Geometry: final body of the model. Coordinates: model frame, mm. Face numbers are marked on the shaded views. A direction names the side the tool comes from. Round coordinates to 2 decimals unless told otherwise and drop trailing zeros. Order: outer loops, then holes, each group sorted by start corner. A loop starts at its lowest first (then second) coordinate and runs counter-clockwise, first axis right, second up. Notation, with made-up numbers: (4, 68) -> (38, 68) arc R18 ccw to (38, 72) -> close; hole circle Ø3 at (73, 59). An arc over 180 degrees is marked (long way). Put each result on its own line as item: value.
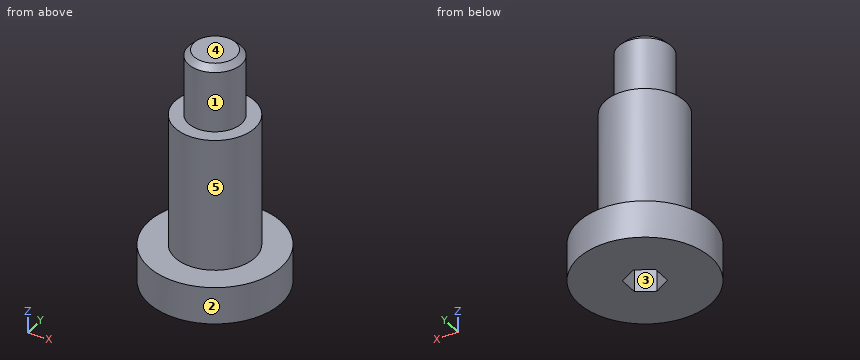
Autodesk Inventor part; units mm, degrees
ref_plane "YZ Plane" through (0, 0, 0) normal (1, 0, 0) x (0, 1, 0)
ref_plane "XZ Plane" through (0, 0, 0) normal (0, 1, 0) x (-1, 0, 0)
ref_plane "XY Plane" through (0, 0, 0) normal (0, 0, 1) x (1, 0, 0)
sketch "Sketch1" plane through (0, 0, 0) normal (0, 1, 0) x (-1, 0, 0)
  line L0 (0, 0) -> (0, 17.8)
  line L1 (0, 17.8) -> (-2, 17.8)
  line L2 (-2, 17.8) -> (-2, 12.8)
  line L3 (-2, 12.8) -> (-3, 12.8)
  line L4 (-3, 12.8) -> (-3, 2.8)
  line L5 (-3, 2.8) -> (-5, 2.8)
  line L6 (-5, 2.8) -> (-5, 0)
  line L7 (-5, 0) -> (0, 0)
  dimension "d0" = 10
  dimension "d1" = 6
  dimension "d2" = 4
  dimension "d3" = 5
  dimension "d4" = 10
  dimension "d5" = 2.8
revolve "Revolution1" add sketch "Sketch1" angle 360 about axis through (0, 0, 0) along (0, 0, 1)
thread "Thread1"
sketch "Sketch2" plane through (0, 0, 0) normal (0, 0, -1) x (-1, 0, 0)
  line L0 (0, 1.4434) -> (1.25, 0.7217)
  line L1 (1.25, 0.7217) -> (1.25, -0.7217)
  line L2 (1.25, -0.7217) -> (0, -1.4434)
  line L3 (0, -1.4434) -> (-1.25, -0.7217)
  line L4 (-1.25, -0.7217) -> (-1.25, 0.7217)
  line L5 (-1.25, 0.7217) -> (0, 1.4434)
  point P0 (0, 0)
  point P1 (0, 0)
  dimension "d9" = 2.5
extrude "Extrusion1" cut sketch "Sketch2" against normal blind 2
chamfer "Chamfer1" distance 0.43 angle 45 1 edges at (-2, 0, 17.8)
properties part number "DBTSY4-10-5-DHC" material "Stainless Steel AISI 304"
1. Cut plane B-B on z = 16.5. Return loops of the section in (x, y).
Ans:
outline: circle Ø4 at (0, 0)
2. Material intervals for probe 1 along Z at (x, y) = (-2.25, -4); probe 2 along Z at (x, y) = (1.5, -1.5); probe 3 along X at (y, z) = (-2, 11), sorted ascending.
Ans:
probe 1: 0 to 2.8
probe 2: 0 to 12.8
probe 3: -2.24 to 2.24
3. Set-up query: the marked faces 1 and 2. Return all of +Z, -Z, +X, -X, +Y, -Y with unobstructed straight access to the full face (end or side cutting, diameter ignored); none if empty.
Ans:
face 1: +Z
face 2: +Z, -Z
4. Cut plane C-C on x = 2.5. Return loops of the section in (y, z), and give its area (3 significant figures).
Ans:
outline: (-4.33, 0) -> (4.33, 0) -> (4.33, 2.8) -> (1.66, 2.8) -> (1.66, 12.8) -> (-1.66, 12.8) -> (-1.66, 2.8) -> (-4.33, 2.8) -> close
area: 57.4 mm²
5. Contact query for flat-ended pins moving along their axis: P1, Ø2, axis at y = 2, z = 9.5, coming from the +X side; P2, Ø4, axis at x = -2, y = -3, coming from the +Z side; P3, Ø3, axis at x = 1.5, z = 13.5, coming from the -Y side (3 decimals). Output: stop coordinate, or through.
Ans:
P1: x = 2.83
P2: z = 17.76
P3: y = -2.995
6. Cut plane A-A on y = 0. Return loops of the section in (x, z).
Ans:
outline: (-5, 0) -> (-1.25, 0) -> (-1.25, 2) -> (1.25, 2) -> (1.25, 0) -> (5, 0) -> (5, 2.8) -> (3, 2.8) -> (3, 12.8) -> (2, 12.8) -> (2, 17.37) -> (1.57, 17.8) -> (-1.57, 17.8) -> (-2, 17.37) -> (-2, 12.8) -> (-3, 12.8) -> (-3, 2.8) -> (-5, 2.8) -> close
7. Cut plane D-D on y = 2.75. Return loops of the section in (x, z).
Ans:
outline: (-4.18, 0) -> (4.18, 0) -> (4.18, 2.8) -> (1.2, 2.8) -> (1.2, 12.8) -> (-1.2, 12.8) -> (-1.2, 2.8) -> (-4.18, 2.8) -> close
8. Draft query along Y for the marked faces 3, 4 and 5. Return one class per face: +Y half, -Y half, draft (parallel to the pull), parting line (faces both ways), or undercut.
Ans:
face 3: undercut
face 4: draft
face 5: parting line
